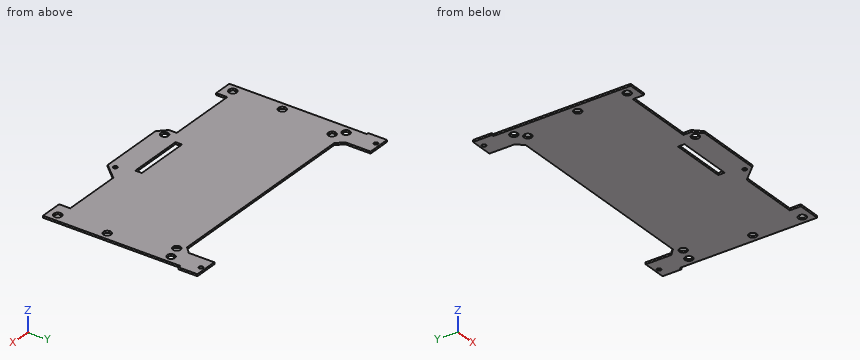
from build123d import *

# Parameters (mm, degrees)
SKETCH1_R           = 3
SKETCH1_R_2         = 1.5
SKETCH1_W           = 43
SKETCH1_H           = 5
BOSS_EXTRUDE1_DEPTH = 1.5


with BuildPart() as part:
    # Sketch1 → Boss-Extrude1 (new body)
    with BuildSketch(Plane.XY):
        Polygon((-100.6, 103), (-83.1, 103), (-83.1, 83.449747468), (-78.150252532, 78.5), (78.950252532, 78.5), (83.9, 83.449747468), (83.9, 103), (101.9, 103), (101.9, 88.5), (99.9, 88.5), (99.9, -17), (82.65, -17), (82.65, -8.5), (36.65, -8.5), (25.9, -20.5), (-25.1, -20.5), (-31.1, -14.5), (-31.1, -8.5), (-85.1, -8.5), (-85.1, -17), (-99.1, -17), (-99.1, 88.5), (-100.6, 88.5), align=None)
        with Locations((93.9, 77)):
            Circle(SKETCH1_R, mode=Mode.SUBTRACT)
        with Locations((83.6, 74)):
            Circle(SKETCH1_R, mode=Mode.SUBTRACT)
        with Locations((93.9, -10)):
            Circle(SKETCH1_R, mode=Mode.SUBTRACT)
        with Locations((93.9, 28)):
            Circle(SKETCH1_R, mode=Mode.SUBTRACT)
        with Locations((93.9, 100)):
            Circle(SKETCH1_R_2, mode=Mode.SUBTRACT)
        with Locations((25.4, -15)):
            Circle(SKETCH1_R_2, mode=Mode.SUBTRACT)
        with Locations((-25.1, -13.5)):
            Circle(SKETCH1_R, mode=Mode.SUBTRACT)
        with Locations((-93.1, -10)):
            Circle(SKETCH1_R, mode=Mode.SUBTRACT)
        with Locations((-93.1, 28)):
            Circle(SKETCH1_R, mode=Mode.SUBTRACT)
        with Locations((-93.1, 77)):
            Circle(SKETCH1_R, mode=Mode.SUBTRACT)
        with Locations((-86.5, 71)):
            Circle(SKETCH1_R, mode=Mode.SUBTRACT)
        with Locations((-93.1, 100)):
            Circle(SKETCH1_R_2, mode=Mode.SUBTRACT)
        Rectangle(SKETCH1_W, SKETCH1_H, mode=Mode.SUBTRACT)
    extrude(amount=BOSS_EXTRUDE1_DEPTH)


solid = part.part
Could you check a few things on this model? Use its own coordinates, in mm. Coordinates: 2 decimals unless noted, no trailing zeros. Write each loop counter-clockwise with the first axis right and the second up, starting at its lowest first coordinate (ties: lowest second). Pieces come first, ordered by that corner, then holes. Notation, with made-up numbers: M 43,75.5 L 75,75.5 A14 ccw 75,89.5 Z; hole C -27,66 d9. An arc over 180 degrees is marked long. One line per question, with ' | ' between items.
1) Imagine slicing it at B-B, the plane y = 28. Write out the boundary of the cut face in (x, z).
Checks:
outline: M -99.1,0 L -96.1,0 L -96.1,1.5 L -99.1,1.5 Z; M -90.1,0 L 90.9,0 L 90.9,1.5 L -90.1,1.5 Z; M 96.9,0 L 99.9,0 L 99.9,1.5 L 96.9,1.5 Z
2) For pin 1 Ø0.8 at (x, z) = (-100, 0.5) entering from -Y, with a flat end and sliding along its axis, tell me the tip position at first contact or that it passes through.
Checks:
pin 1: y = 88.5
3) Imagine slicing it at C-C, the plane x = 62. Write out the boundary of the cut face in (y, z), and give its area (4 significant figures).
Checks:
outline: M -8.5,0 L 78.5,0 L 78.5,1.5 L -8.5,1.5 Z | area: 130.5 mm²
4) Imagine slicing it at A-A, the plane y = 93. Write out the boundary of the cut face in (x, z).
Checks:
outline: M -100.6,0 L -83.1,0 L -83.1,1.5 L -100.6,1.5 Z; M 83.9,0 L 101.9,0 L 101.9,1.5 L 83.9,1.5 Z
5) Imagine slicing it at D-D, the plane z = 0.6. Give the number of separate pieces and of enclosed holes in the cut face, and give its area (3 significant figures).
Checks:
separate pieces: 1 | enclosed holes: 13 | area: 18,700 mm²
6) I need wall thicknesses on probe 1 along Y at (x, z) = (93.9, 0.75); probe 2 along Y at (x, z) = (25.4, 0.4); probe 3 along X at (y, z) = (100, 0.4). Which ranges of each line are inside material? Lowest first, please. Write a range as [from, to].
Checks:
probe 1: [-17, -13], [-7, 25], [31, 74], [80, 98.5], [101.5, 103] | probe 2: [-20.5, -16.5], [-13.5, 78.5] | probe 3: [-100.6, -94.6], [-91.6, -83.1], [83.9, 92.4], [95.4, 101.9]
